```python
from build123d import *

# Parameters (mm, degrees)
F0_R     = 1.65
F0_W     = 16.5
F0_H     = 7
F1_DEPTH = 4
F2_SIZE  = 1.75


with BuildPart() as f1:
    # F0 (on Top) → F1 (new body)
    with BuildSketch(Plane.XY):
        with BuildLine():
            Line((10.478546, -5.5), (14.5, -5.5))
            Line((14.5, -5.5), (14.5, 3.75))
            Line((14.5, 3.75), (9.5, 3.75))
            Line((9.5, 3.75), (9.5, 5.5))
            Line((9.5, 5.5), (-9.5, 5.5))
            Line((-9.5, 5.5), (-9.5, 3.75))
            Line((-9.5, 3.75), (-14.5, 3.75))
            Line((-14.5, 3.75), (-14.5, -5.5))
            Line((-14.5, -5.5), (-10.478546, -5.5))
            ThreePointArc((-10.478546, -5.5), (0, -7.681161), (10.478546, -5.5))
        make_face()
        with Locations((-12, 0)):
            Circle(F0_R, mode=Mode.SUBTRACT)
        with Locations((0, -1)):
            Rectangle(F0_W, F0_H, mode=Mode.SUBTRACT)
        with Locations((12, 0)):
            Circle(F0_R, mode=Mode.SUBTRACT)
    extrude(amount=F1_DEPTH)

    # F2
    f2_edges = [f1.edges().sort_by_distance(p)[0] for p in [
        (0, 5.5, 4),
    ]]
    chamfer(f2_edges, length=F2_SIZE)


solid = f1.part
```
Verification items for the finished model (mm, model axes). A direction names the side the tool comes from. Round coordinates to 2 decimals unless told otherwise and drop trailing zeros. Write each loop counter-clockwise with the first axis right and the second up, starting at its lowest first coordinate (ties: lowest second). Pieces come first, ordered by that corner, then holes.
1. Scan lines: L1, parallel to X at y = 1.75, z = 2.45; L2, parallel to Y at x = -12, z = 1.55; L3, parallel to X at y = 0.25, z = 3.2. Record each from-to range of solid material in increasing order.
2. Gauge pin test, flat ends, axial feed: P1, Ø2, axis at x = 13.5, z = 2.5, coming from the -Y side; P2, Ø0.9, axis at y = 5, z = 2, coming from the -X side; P3, Ø0.5, axis at y = 4.5, z = 3, coming from the +X side. Record the tip position at first contact, or that the pin passes through.
3. Access from +Z, -Z, +X, -X, +Y, -Y to the whole of each face (thin tool, end or side, straight path). Record for faces 1 (the flat face through (12, 3.75, 2)), 2 (the flat face through (0, 2.5, 2)), 3 (the flat face through (-12, 3.75, 2)), 4 (the flat face through (-13, -5.5, 2)), 5 (the flat face through (12, -5.5, 2)).
4. Section check A-A on x = 12. Enter the section's corners in (y, z), plus the area to 3 significant figures.
5. Section check B-B on z = 0.8. Enter the section's corners in (x, y).
6. Section check D-D on y = -2. Enter the section's corners in (x, z).
7. Section check C-C on y = 0. Enter the section's corners in (x, z), plus the area to 3 significant figures.
8. Draft check along X on faces 6 (the flat face through (0, -4.5, 2)), 7 (the flat face through (9.5, 5, 2)), 8 (the flat face through (0, 5.5, 1)). Enter one of: +X half, -X half, draft (parallel to the pull), parting line (faces both ways), or undercut.
Answer:
1. L1: x = -14.5 to -8.25, 8.25 to 14.5
1. L2: y = -5.5 to -1.65, 1.65 to 3.75
1. L3: x = -14.5 to -13.63, -10.37 to -8.25, 8.25 to 10.37, 13.63 to 14.5
2. P1: stops at y = -5.5
2. P2: stops at x = -9.5
2. P3: stops at x = 9.5
3. face 1: +Z, -Z, +X, +Y
3. face 2: +Z, -Z
3. face 3: +Z, -Z, -X, +Y
3. face 4: +Z, -Z, -X, -Y
3. face 5: +Z, -Z, +X, -Y
4. outline: (-5.5, 0) - (-1.65, 0) - (-1.65, 4) - (-5.5, 4) - close; (1.65, 0) - (3.75, 0) - (3.75, 4) - (1.65, 4) - close
4. area: 23.8 mm2
5. outline: (-14.5, -5.5) - (-10.48, -5.5) arc R26.26 ccw to (10.48, -5.5) - (14.5, -5.5) - (14.5, 3.75) - (9.5, 3.75) - (9.5, 5.5) - (-9.5, 5.5) - (-9.5, 3.75) - (-14.5, 3.75) - close; hole circle Ø3.3 at (-12, 0); hole (-8.25, -4.5) - (8.25, -4.5) - (8.25, 2.5) - (-8.25, 2.5) - close; hole circle Ø3.3 at (12, 0)
6. outline: (-14.5, 0) - (-8.25, 0) - (-8.25, 4) - (-14.5, 4) - close; (8.25, 0) - (14.5, 0) - (14.5, 4) - (8.25, 4) - close
7. outline: (-14.5, 0) - (-13.65, 0) - (-13.65, 4) - (-14.5, 4) - close; (-10.35, 0) - (-8.25, 0) - (-8.25, 4) - (-10.35, 4) - close; (8.25, 0) - (10.35, 0) - (10.35, 4) - (8.25, 4) - close; (13.65, 0) - (14.5, 0) - (14.5, 4) - (13.65, 4) - close
7. area: 23.6 mm2
8. face 6: undercut
8. face 7: +X half
8. face 8: draft
